The figure shows three views and two pictorial views of one solid part (mm, origin at its lowest corner). Answer the questions. A direction names the side the tool comes from. Round coordinates to 2 decimals unless told otherwise and drop trailing zeros. Loops run counter-clockwise (first coordinate to the right, second up) from the corner with the lowest first, then second, coordinate; pieces in that order, holes last. Notation, with made-up numbers: (-12.75, 68.25) -> (1.25, 68.25) arc R25 cw to (1.25, 105.25) -> close; hole circle Ø6 at (64, 24.25). An arc over 180 degrees is marked (long way). Put each result on its own line as item: value.
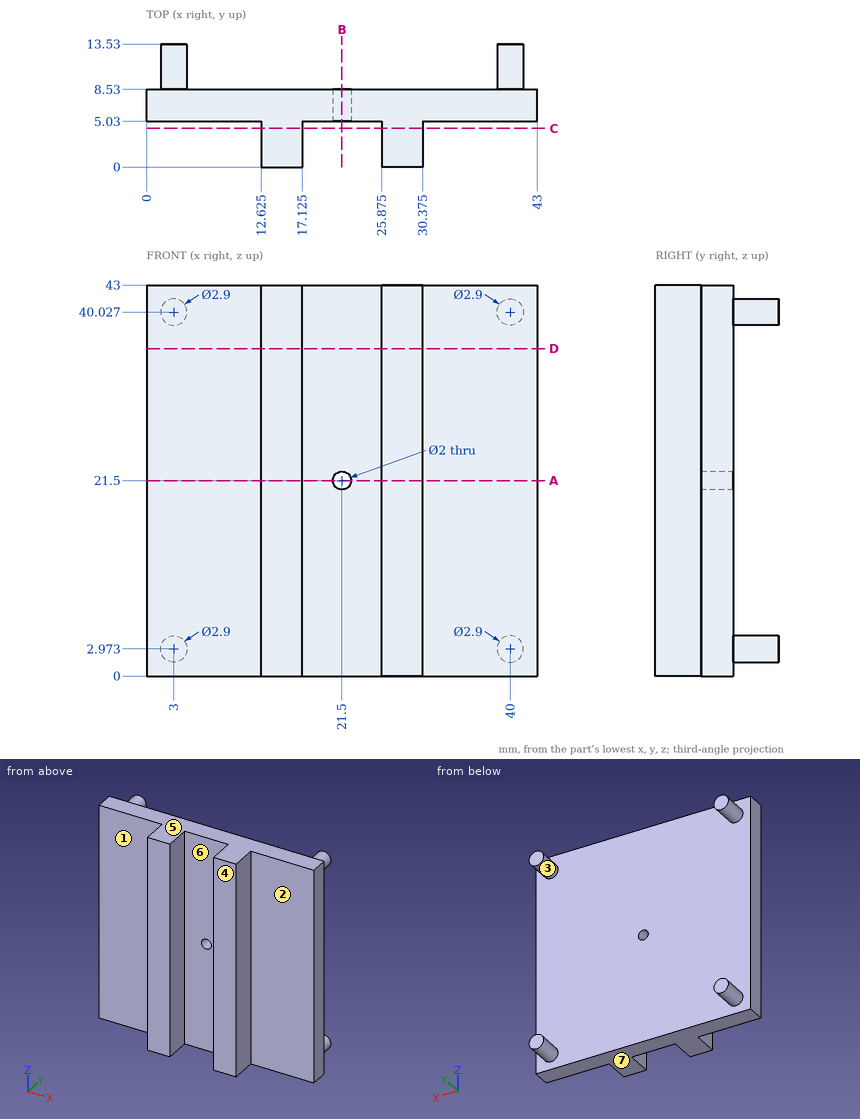
Item 1: The part is cut by section C-C (y = 4.25). Determine the outline of the cut face in (x, z) (3 decimals), then the cut area to 3 significant figures.
Derived:
outline: (12.625, 0) -> (17.125, 0) -> (17.125, 43) -> (12.625, 43) -> close; (25.875, 0) -> (30.375, 0) -> (30.375, 43) -> (25.875, 43) -> close
area: 387 mm^2
Item 2: The part is cut by section B-B (x = 21.5). Determine the outline of the cut face in (y, z), then the cut area to 4 significant figures.
Derived:
outline: (5.03, 0) -> (8.53, 0) -> (8.53, 20.5) -> (5.03, 20.5) -> close; (5.03, 22.5) -> (8.53, 22.5) -> (8.53, 43) -> (5.03, 43) -> close
area: 143.5 mm^2
Item 3: Find the intervals of material crossed by line 1 along X through (y, z) = (1.25, 18.5) (3 decimals); line 2 along X through (y, z) = (7.75, 21.5); line 3 along Y through (x, z) = (5.5, 5.5), in increasing order.
Derived:
line 1: x = 12.625 to 17.125, 25.875 to 30.375
line 2: x = 0 to 20.5, 22.5 to 43
line 3: y = 5.03 to 8.53
Item 4: Which of the six approach directions +Z, -Z, +X, -X, +Y, -Y give full straight-line access (tool end or side, diameter ignored) to the marked faces 1, 2, 3, 4 and 5?
Derived:
face 1: +Z, -Z, -X, -Y
face 2: +Z, -Z, +X, -Y
face 3: +Y
face 4: +Z, -Z, +X, -X, -Y
face 5: +Z, +X, -X, +Y, -Y
Item 5: The part is cut by section D-D (z = 36). Determine the outline of the cut face in (x, y) (3 decimals), then the cut area to 3 significant figures.
Derived:
outline: (0, 5.03) -> (12.625, 5.03) -> (12.625, 0) -> (17.125, 0) -> (17.125, 5.03) -> (25.875, 5.03) -> (25.875, 0) -> (30.375, 0) -> (30.375, 5.03) -> (43, 5.03) -> (43, 8.53) -> (0, 8.53) -> close
area: 196 mm^2
Item 6: The part is cut by section A-A (z = 21.5). Determine the outline of the cut face in (x, y) (3 decimals).
Derived:
outline: (0, 5.03) -> (12.625, 5.03) -> (12.625, 0) -> (17.125, 0) -> (17.125, 5.03) -> (20.5, 5.03) -> (20.5, 8.53) -> (0, 8.53) -> close; (22.5, 5.03) -> (25.875, 5.03) -> (25.875, 0) -> (30.375, 0) -> (30.375, 5.03) -> (43, 5.03) -> (43, 8.53) -> (22.5, 8.53) -> close
Item 7: For a pull along X with two mould halves and no side action, classify the marked faces 6 and 7 as pulls with the +X half, pulls with the -X half, needs draft (parallel to the pull), parting line crosses it, or undercut.
Derived:
face 6: undercut
face 7: needs draft
Item 8: Flat-ended cylindrical pins translate along their axes: pin 1 Ø12 at (x, z) = (28, 28.5) entering from +Y; pin 2 Ø1 at (y, z) = (3.5, 19.5) entering from -X (3 decimals); pin 3 Ø2.5 at (y, z) = (3, 30) entering from +X (3 decimals); pin 4 Ø3 at (y, z) = (11, 12.5) entering from -X. Find the tip coordinate at first contact, or state that the pin passes through.
Derived:
pin 1: stops at y = 8.53
pin 2: stops at x = 12.625
pin 3: stops at x = 30.375
pin 4: passes through
